Geometry check sheet. Reference: the model listing, model coordinates, mm. A direction names the side the tool comes from. Round coordinates to 2 decimals unless told otherwise and drop trailing zeros. Write each loop counter-clockwise with the first axis right and the second up, starting at its lowest first coordinate (ties: lowest second). Pieces come first, ordered by that corner, then holes. Notation, with made-up numbers: M 58.25,34 L 65.25,34 A17 ccw 65.25,65 Z; hole C -27,50 d9. An arc over 180 degrees is marked long. Use a Markdown table: item, result.
```python
from build123d import *

# Parameters (mm, degrees)
SKETCH1_W           = 40
SKETCH1_H           = 19.58331309
BOSS_EXTRUDE1_DEPTH = 25
CUT_EXTRUDE1_REACH  = 306.991
SKETCH2_R           = 12.5


with BuildPart() as part:
    # Sketch1 → Boss-Extrude1 (new, symmetric)
    with BuildSketch(Plane(origin=(0, 0, 0), x_dir=(0, 0, -1), z_dir=(1, 0, 0))):
        Polygon((-25, -150), (-25, 150), (25, 150), (25, -150), (25, -152.934399054), (20, -152.934399054), (20, -150), (20, -128.351099054), (-18.690995821, -152.129907993), (-20, -152.934399054), (-25, -152.934399054), align=None)
        Polygon((15.225378118, 120.41668691), (-20, 120.41668691), (-20, 98.767785964), align=None, mode=Mode.SUBTRACT)
        Polygon((-20, -147.065600946), (-20, -103.767412144), (15.225406311, -125.416682672), align=None, mode=Mode.SUBTRACT)
        Polygon((-20, -97.898614036), (-20, -54.600812144), (15.225378116, -76.250065344), align=None, mode=Mode.SUBTRACT)
        with Locations((-3.9301e-05, 135.208343455)):
            Rectangle(SKETCH1_W, SKETCH1_H, mode=Mode.SUBTRACT)
        Polygon((20, -73.315687856), (20, -30.017885964), (-15.225378116, -51.666434656), align=None, mode=Mode.SUBTRACT)
        Polygon((15.225378116, 71.249734656), (-20, 92.898987856), (-20, 49.601185964), align=None, mode=Mode.SUBTRACT)
        Polygon((15.225378116, 22.083134656), (-20, 43.732387856), (-20, 0.434585964), align=None, mode=Mode.SUBTRACT)
        Polygon((15.225378116, -27.083465344), (-20, -5.434212144), (-20, -48.732014036), align=None, mode=Mode.SUBTRACT)
        Polygon((-15.225378116, 95.833365344), (20, 117.481914036), (20, 74.184112144), align=None, mode=Mode.SUBTRACT)
        Polygon((-15.225378116, 46.666765344), (20, 68.315314036), (20, 25.017512144), align=None, mode=Mode.SUBTRACT)
        Polygon((-15.225378116, -2.499834656), (20, 19.148714036), (20, -24.149087856), align=None, mode=Mode.SUBTRACT)
        Polygon((20, -79.184485964), (-15.225378116, -100.833034656), (20, -122.482287856), align=None, mode=Mode.SUBTRACT)
    extrude(amount=BOSS_EXTRUDE1_DEPTH, both=True)

    # Sketch2 → Cut-Extrude1 (cut, up to next)
    with BuildSketch(Plane(origin=(0, 150, 0), x_dir=(1, 0, 0), z_dir=(0, 1, 0)), mode=Mode.PRIVATE) as cut_extrude1_sk1:
        with Locations(Location((0, 0, 0), (0, 0, 270))):
            Circle(SKETCH2_R)
    cut_extrude1_tool1 = extrude(cut_extrude1_sk1.sketch, amount=-CUT_EXTRUDE1_REACH, mode=Mode.PRIVATE) & part.part
    add(cut_extrude1_tool1.solids().sort_by_distance((0, 150, 0))[0], mode=Mode.SUBTRACT)


solid = part.part
```
Item 1: Go/stop test with flat-tipped pins: pin 1 (1.5 mm diameter, centred on y = -117.5, z = -17, fed in from -X); pin 2 (22.5 mm diameter, centred on x = 0, z = 0, fed in from +Y); pin 3 (4 mm diameter, centred on x = 16.5, z = 13.5, fed in from -Y); pin 4 (12 mm diameter, centred on x = -9, z = 0.5, fed in from +Y). Record where each tip stops, or that it passes through.
Outcome:
| item | result |
|---|---|
| pin 1 | passes through |
| pin 2 | stops at y = 125.42 |
| pin 3 | stops at y = -150.17 |
| pin 4 | stops at y = 150 |
Item 2: Material ranges on line 1 along X through (y, z) = (146.35, 0); line 2 along Z through (x, y) = (1.5, 85); line 3 along Z through (x, y) = (9, -72), recorded low to high. Write a range as from..to.
Outcome:
| item | result |
|---|---|
| line 1 | x = -25..-12.5, 12.5..25 |
| line 2 | z = -25..-20, -2.4..7.15, 20..25 |
| line 3 | z = -25..-20, -17.86..-8.31, 20..25 |
Item 3: Access from +Z, -Z, +X, -X, +Y, -Y to the whole of each face (thin tool, end or side, straight path). Record for faces 4 (the face through (11.5, 150, 5.9)), 5 (the face through (0.35, -40.691, -2.634)).
Outcome:
| item | result |
|---|---|
| face 4 | +Z, -Z, +X, -X, +Y |
| face 5 | +X, -X |
Item 4: Mould release check, pull along Y, two halves, no side actions. Record for faces 1 (the face through (0, -77, 20)), 2 (the face through (0, -152.934, -23)), 3 (the face through (0, 1, 25)): +Y half, -Y half, draft (parallel to the pull), parting line (faces both ways), or undercut.
Outcome:
| item | result |
|---|---|
| face 1 | undercut |
| face 2 | -Y half |
| face 3 | draft |
Item 5: Cross-section at A-A, the plane y = -84.5. Record the cut outline in (x, z).
Outcome:
| item | result |
|---|---|
| outline | M -25,-25 L 25,-25 L 25,-20 L -25,-20 Z; M -25,-11.35 L 25,-11.35 L 25,-1.8 L -25,-1.8 Z; M -25,20 L 25,20 L 25,25 L -25,25 Z |
Item 6: Cross-section at B-B, the plane x = -15. Count the separate pieces of the cut face and the enclosed holes in it, and give its area (3 significant figures).
Outcome:
| item | result |
|---|---|
| separate pieces | 1 |
| enclosed holes | 12 |
| area | 5,860 mm2 |
